Read the model definition and answer for the solid it produces. Units are mm, in the model's axes. A direction names the side the tool comes from. Coordinates: 2 decimals unless noted, no trailing zeros. Write each loop counter-clockwise with the first axis right and the second up, starting at its lowest first coordinate (ties: lowest second). Pieces come first, ordered by that corner, then holes. Notation, with made-up numbers: (6.5, 39.5) -> (55.5, 39.5) arc R15 cw to (55.5, 68.5) -> close; hole circle Ø1 at (66.25, -0.5). An arc over 180 degrees is marked (long way). Write item = value, one per line. Start each with the question number.
1) Find the intervals of material crossed by line 1 along X through (y, z) = (-2.25, 15.5); line 2 along Z through (x, y) = (15, -3); line 3 along X through (y, z) = (-2.5, 16.5), in increasing order. Write a range as from..to.
2) Section B-B (y = -12) is taken. Determine the outline of the cut face in (x, z).
3) Section C-C (x = -15) is taken. Determine the outline of the cut face in (y, z).
4) A tool of negligible diameter and unlimited length cuts with its end or side. For faces 3 (the face through (-0.28, -12.67, 3.7)), 4 (the face through (-0.247, -35.951, -11.247)), 5 (the face through (0, -30.5, 3)), 6 (the face through (0, -21, 12)), from which of +Z, -Z, +X, -X, +Y, -Y can it reach the whole face along a straight path? Write none if from no direction.
5) Flat-ended cylindrical pins translate along their axes: pin 1 Ø4 at (x, z) = (-10, 16.5) entering from -Y; pin 2 Ø4 at (x, y) = (11.5, -27.5) entering from +Z; pin 3 Ø15.5 at (x, z) = (-2.5, 6.5) entering from -Y. Find the tip coordinate at first contact, or state that the pin passes through.
6) Section D-D (x = 3) is taken. Determine the outline of the cut face in (y, z).
7) Section A-A (y = -36) is taken. Determine the outline of the cut face in (x, z).
8) For a pull along X with two mould halves and no side action, classify faces 1 (the face through (0, -25, -12.5)), 2 (the face through (13.926, -4.31, 15.004)) as released by +X, released by -X, zero draft, split by the parting line, or undercut.
from build123d import *

# Parameters (mm, degrees)
SKETCH1_W             = 40
SKETCH1_H             = 40
BOSS_EXTRUDE1_DEPTH   = 41
M4X0_7_TAPPED_HOLE1_D = 3.3
SKETCH11_W            = 11.25
SKETCH11_H            = 7
CUT_EXTRUDE5_REACH    = 43
SKETCH12_R            = 10
M4X0_7_TAPPED_HOLE2_D = 3.3
SKETCH15_W            = 40
SKETCH15_H            = 7.5
CUT_EXTRUDE6_DEPTH    = 32.5
SKETCH16_W            = 22.5
SKETCH16_H            = 7
CUT_EXTRUDE7_DEPTH    = 21
CUT_EXTRUDE8_REACH    = 43
SKETCH17_W            = 22.5
SKETCH17_H            = 12.5
CUT_EXTRUDE9_DEPTH    = 2
CUT_EXTRUDE10_DEPTH   = 41
SKETCH20_W            = 22.5
SKETCH20_H            = 10
CUT_EXTRUDE11_DEPTH   = 12.5
SKETCH21_W            = 0.5
SKETCH21_H            = 32.5
CUT_EXTRUDE12_DEPTH   = 41


with BuildPart() as part:
    # Sketch1 → Boss-Extrude1 (new body)
    with BuildSketch(Plane(origin=(0, 0, 0), x_dir=(1, 0, 0), z_dir=(0, 1, 0))):
        Rectangle(SKETCH1_W, SKETCH1_H)
    extrude(amount=-BOSS_EXTRUDE1_DEPTH)

    # M4x0.7 Tapped Hole1 (through all)
    with Locations(Plane(origin=(0, 0, 0), x_dir=(1, 0, 0), z_dir=(0, 1, 0))):
        with Locations((-15.5, 15.5), (15.5, 15.5), (15.5, -15.5), (-15.5, -15.5)):
            Hole(M4X0_7_TAPPED_HOLE1_D / 2)

    # Sketch11 → Cut-Revolve2 (revolve, cut)
    with BuildSketch(Plane.XY):
        with Locations((5.625, -36)):
            Rectangle(SKETCH11_W, SKETCH11_H)
    revolve(axis=Axis((0, 0, 0), (0, -1, 0)), mode=Mode.SUBTRACT)

    # Sketch12 → Cut-Extrude5 (cut, up to next)
    with BuildSketch(Plane.XZ.offset(41), mode=Mode.PRIVATE) as cut_extrude5_sk1:
        Circle(SKETCH12_R)
    cut_extrude5_tool1 = extrude(cut_extrude5_sk1.sketch, amount=-CUT_EXTRUDE5_REACH, mode=Mode.PRIVATE) & part.part
    add(cut_extrude5_tool1.solids().sort_by_distance((0, -41, 0))[0], mode=Mode.SUBTRACT)

    # M4x0.7 Tapped Hole2 (through all)
    with Locations(Plane(origin=(0, 0, -20), x_dir=(-1, 0, 0), z_dir=(0, 0, -1))):
        with Locations((15, -36), (-15, -36)):
            Hole(M4X0_7_TAPPED_HOLE2_D / 2)

    # Sketch15 → Cut-Extrude6 (cut)
    with BuildSketch(Plane.XZ.offset(41)):
        with Locations((0, -16.25)):
            Rectangle(SKETCH15_W, SKETCH15_H)
        with Locations((0, 16.25)):
            Rectangle(SKETCH15_W, SKETCH15_H)
    extrude(amount=-CUT_EXTRUDE6_DEPTH, mode=Mode.SUBTRACT)

    # Sketch16 → Cut-Extrude7 (cut, through all)
    with BuildSketch(Plane.XY):
        with Locations((0, -36)):
            Rectangle(SKETCH16_W, SKETCH16_H)
    extrude(amount=CUT_EXTRUDE7_DEPTH, mode=Mode.SUBTRACT)

    # Sketch17 → Cut-Extrude8 (cut, up to next)
    with BuildSketch(Plane.XZ.offset(41), mode=Mode.PRIVATE) as cut_extrude8_sk1:
        with Locations((0, 6.25)):
            Rectangle(SKETCH17_W, SKETCH17_H)
    cut_extrude8_tool1 = extrude(cut_extrude8_sk1.sketch, amount=-CUT_EXTRUDE8_REACH, mode=Mode.PRIVATE) & part.part
    add(cut_extrude8_tool1.solids().sort_by_distance((0, -41, 6.25))[0], mode=Mode.SUBTRACT)

    # Sketch18 → Cut-Extrude9 (cut)
    with BuildSketch(Plane.XZ.offset(32.5)):
        with BuildLine():
            Line((-7, 0), (-7, 12.5))
            Line((-7, 12.5), (7, 12.5))
            Line((7, 12.5), (7, 0))
            ThreePointArc((7, 0), (0, -7), (-7, 0))
        make_face()
    extrude(amount=-CUT_EXTRUDE9_DEPTH, mode=Mode.SUBTRACT)

    # Sketch19 → Cut-Extrude10 (cut, through all)
    with BuildSketch(Plane.ZY.offset(20)):
        Polygon((0, -25), (7.5, 0), (-7.5, 0), align=None)
    extrude(amount=-CUT_EXTRUDE10_DEPTH, mode=Mode.SUBTRACT)

    # Sketch20 → Cut-Extrude11 (cut)
    with BuildSketch(Plane.XY.offset(12.5)):
        with Locations((0, -36)):
            Rectangle(SKETCH20_W, SKETCH20_H)
    extrude(amount=-CUT_EXTRUDE11_DEPTH, mode=Mode.SUBTRACT)

    # Sketch21 → Cut-Extrude12 (cut, through all)
    with BuildSketch(Plane.ZY.offset(20)):
        with Locations((12.25, -24.75)):
            Rectangle(SKETCH21_W, SKETCH21_H)
    extrude(amount=-CUT_EXTRUDE12_DEPTH, mode=Mode.SUBTRACT)


solid = part.part
Answer key:
q1.line_1 = -20..-17.15, -13.85..13.85, 17.15..20
q1.line_2 = -20..-17.07, -13.93..-6.6, 6.6..13.93, 17.07..20
q1.line_3 = -20..-16.81, -14.19..14.19, 16.81..20
q2.outline = (-20, -12.5) -> (20, -12.5) -> (20, -3.9) -> (-20, -3.9) -> close; (-20, 3.9) -> (20, 3.9) -> (20, 12) -> (-20, 12) -> close
q3.outline = (-41, -12.5) -> (-37.65, -12.5) -> (-37.65, 12) -> (-41, 12) -> close; (-34.35, -12.5) -> (-8.5, -12.5) -> (-8.5, -13.93) -> (0, -13.93) -> (0, -7.5) -> (-25, 0) -> (0, 7.5) -> (0, 13.93) -> (-8.5, 13.93) -> (-8.5, 12) -> (-34.35, 12) -> close; (-8.5, -20) -> (0, -20) -> (0, -17.07) -> (-8.5, -17.07) -> close; (-8.5, 17.07) -> (0, 17.07) -> (0, 20) -> (-8.5, 20) -> close
q4.face_3 = +X, -X, +Y
q4.face_4 = +Z
q4.face_5 = +Z, -Y
q4.face_6 = +Z, +X, -X, -Y
q5.pin_1 = -8.5
q5.pin_2 = 12
q5.pin_3 = -31
q6.outline = (-41, -12.5) -> (-8.5, -12.5) -> (-8.5, -20) -> (0, -20) -> (0, -7.5) -> (-25, 0) -> (0, 7.5) -> (0, 20) -> (-8.5, 20) -> (-8.5, 12) -> (-30.5, 12) -> (-30.5, -6.32) -> (-32.5, -6.32) -> (-32.5, -10.84) -> (-39.5, -10.84) -> (-39.5, -9.54) -> (-41, -9.54) -> close
q7.outline = (-20, -12.5) -> (-16.65, -12.5) -> (-16.65, 12) -> (-20, 12) -> close; (-13.35, -12.5) -> (13.35, -12.5) -> (13.35, 12) -> (11.25, 12) -> (11.25, 0) arc R11.25 cw to (-11.25, 0) -> (-11.25, 12) -> (-13.35, 12) -> close; (16.65, -12.5) -> (20, -12.5) -> (20, 12) -> (16.65, 12) -> close
q8.face_1 = zero draft
q8.face_2 = undercut
